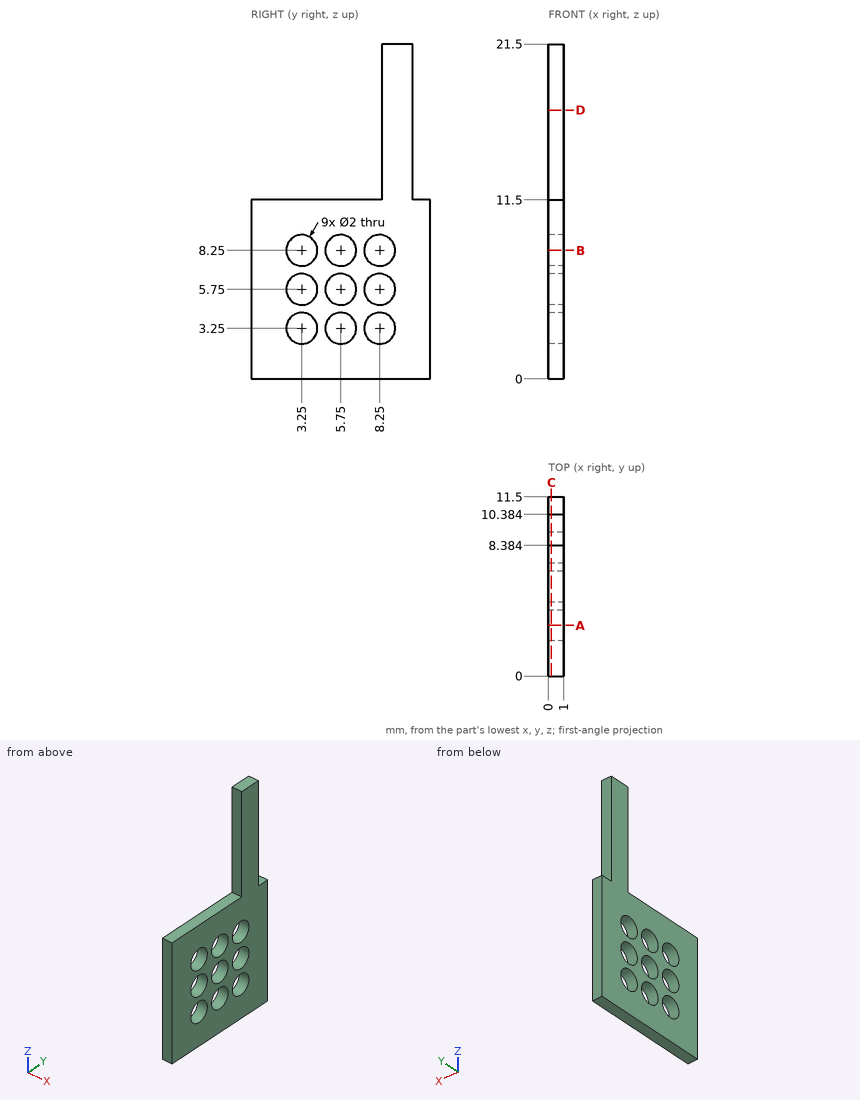
For this review, use the dimensioned drawing (mm, ordinates from the lowest corner) and the shaded views. Round coordinates to 2 decimals unless told otherwise and drop trailing zeros. Order: outer loops, then holes, each group sorted by start corner. A loop starts at its lowest first (then second) coordinate and runs counter-clockwise, first axis right, second up.
1) Consider section C-C (x = 0.2). Count the separate pieces of the cut face and the enclosed holes in it, plus the area to 3 significant figures.
The answers:
separate pieces: 1
enclosed holes: 9
area: 124 mm2
2) Consider section D-D (z = 17.25). State the section outline as (x, y) points.
The answers:
outline: (0, 8.38) - (1, 8.38) - (1, 10.38) - (0, 10.38) - close
3) Consider section A-A (y = 3.25). State the section outline as (x, z) points.
The answers:
outline: (0, 0) - (1, 0) - (1, 2.25) - (0, 2.25) - close; (0, 4.25) - (1, 4.25) - (1, 4.75) - (0, 4.75) - close; (0, 6.75) - (1, 6.75) - (1, 7.25) - (0, 7.25) - close; (0, 9.25) - (1, 9.25) - (1, 11.5) - (0, 11.5) - close
4) Clearance check with flat-ended pins moving along their axes: pin 1 Ø0.5 at (x, z) = (0.5, 16.5) entering from -Y; pin 2 Ø0.5 at (x, y) = (0.5, 6) entering from +Z; pin 3 Ø2.5 at (y, z) = (8.25, 3.25) entering from +X. State where each tip first meets the part, or that it passes through.
The answers:
pin 1: stops at y = 8.38
pin 2: stops at z = 11.5
pin 3: stops at x = 1
5) For L1, parallel to Z at x = 0.6, y = 5.75; L2, parallel to Z at x = 0.65, y = 2.75; L3, parallel to Y at x = 0.3, z = 9, list the stretches that pass through material, from the lowest coordinate up.
The answers:
L1: z = 0 to 2.25, 4.25 to 4.75, 6.75 to 7.25, 9.25 to 11.5
L2: z = 0 to 2.38, 4.12 to 4.88, 6.62 to 7.38, 9.12 to 11.5
L3: y = 0 to 2.59, 3.91 to 5.09, 6.41 to 7.59, 8.91 to 11.5
